Can you work these out from the model? Positions are in its coordinate system, mm. Round coordinates to 2 decimals unless told otherwise and drop trailing zeros. Loops run counter-clockwise (first coordinate to the right, second up) from the corner with the lowest first, then second, coordinate; pieces in that order, holes last. Notation, with made-up numbers: (-25.75, 35.5) - (-10.75, 35.5) arc R21 cw to (-10.75, 47.5) - close; hole circle Ø7 at (-26.75, 42). An arc over 180 degrees is marked (long way). Answer as CSV lines item,"result".
```python
from build123d import *

# Parameters (mm, degrees)
SKETCH1_W           = 14
SKETCH1_H           = 14
BOSS_EXTRUDE2_DEPTH = 1.2
FILLET1_R           = 1
CUT_EXTRUDE2_REACH  = 3.2
SKETCH2_R           = 2.2


with BuildPart() as part:
    # Sketch1 → Boss-Extrude2 (new body)
    with BuildSketch(Plane.XY):
        with BuildLine():
            Line((81.33, -202.9), (79.33, -202.9))
            Line((79.33, -202.9), (76.73, -202.9))
            Line((76.73, -202.9), (76.73, -212.03))
            Line((76.73, -212.03), (76.73, -283.1))
            Line((76.73, -283.1), (79.4, -283.1))
            Line((79.4, -283.1), (81.33, -283.1))
            Line((81.33, -283.1), (81.33, -270.169))
            Line((81.33, -270.169), (95.33, -270.169))
            Line((95.33, -270.169), (95.33, -284.169))
            Line((95.33, -284.169), (81.6, -284.169))
            Line((81.6, -284.169), (81.6, -285.300000001))
            Line((81.6, -285.300000001), (81.6, -288.000000001))
            Line((81.6, -288.000000001), (104.85, -288.000000001))
            Line((104.85, -288.000000001), (113.94, -288.000000001))
            Line((113.94, -288.000000001), (133.73, -288.000000001))
            Line((133.73, -288.000000001), (136.73, -285.000000001))
            Line((136.73, -285.000000001), (152.86, -285.000000001))
            Line((152.86, -285.000000001), (161.94, -285.000000001))
            Line((161.94, -285.000000001), (178.73, -285.000000001))
            Line((178.73, -285.000000001), (195.659492, -289.51666))
            Line((195.659492, -289.51666), (208.778384908, -297.081045818))
            Line((208.778384908, -297.081045818), (210.094127263, -294.801069106))
            Line((210.094127263, -294.801069106), (210.094924986, -294.799686776))
            ThreePointArc((210.094924986, -294.799686776), (211.43094748, -293.774869597), (213.100313224, -293.994924986))
            Line((213.100313224, -293.994924986), (215.397829273, -295.321900182))
            Line((215.397829273, -295.321900182), (225.98, -277))
            Line((225.98, -277), (225.98, -256.415))
            Line((225.98, -256.415), (225.98, -247.025))
            Line((225.98, -247.025), (225.98, -214.605))
            Line((225.98, -214.605), (225.98, -205.215))
            Line((225.98, -205.215), (225.98, -197))
            ThreePointArc((225.98, -197), (224.515534, -193.464466), (220.98, -192))
            Line((220.98, -192), (206.7, -192))
            Line((206.7, -192), (206.7, -194.6))
            ThreePointArc((206.7, -194.6), (204.5, -196.8), (202.3, -194.6))
            Line((202.3, -194.6), (202.3, -192))
            Line((202.3, -192), (179.02, -192))
            Line((179.02, -192), (169.96, -192))
            Line((169.96, -192), (136.73, -192))
            Line((136.73, -192), (133.73, -192))
            Line((133.73, -192), (127.73, -198))
            Line((127.73, -198), (108.89, -198))
            Line((108.89, -198), (99.78, -198))
            Line((99.78, -198), (82.73, -198))
            Line((82.73, -198), (81.53, -198))
            Line((81.53, -198), (81.53, -200.7))
            Line((81.53, -200.7), (81.53, -201.794))
            Line((81.53, -201.794), (95.33, -201.794))
            Line((95.33, -201.794), (95.33, -215.794))
            Line((95.33, -215.794), (81.33, -215.794))
            Line((81.33, -215.794), (81.33, -202.9))
        make_face()
        with Locations((106.43, -277.169)):
            Rectangle(SKETCH1_W, SKETCH1_H, mode=Mode.SUBTRACT)
        with Locations((124.53, -277.169)):
            Rectangle(SKETCH1_W, SKETCH1_H, mode=Mode.SUBTRACT)
        with Locations((88.33, -260.094)):
            Rectangle(SKETCH1_W, SKETCH1_H, mode=Mode.SUBTRACT)
        with Locations((106.43, -260.094)):
            Rectangle(SKETCH1_W, SKETCH1_H, mode=Mode.SUBTRACT)
        with Locations((124.53, -260.094)):
            Rectangle(SKETCH1_W, SKETCH1_H, mode=Mode.SUBTRACT)
        with Locations((142.63, -255.362582)):
            Rectangle(SKETCH1_W, SKETCH1_H, mode=Mode.SUBTRACT)
        with Locations((168.416577, -274.987582)):
            Rectangle(SKETCH1_W, SKETCH1_H, mode=Mode.SUBTRACT)
        Polygon((194.375574468, -286.3230671), (180.8526129, -282.699600468), (184.476079532, -269.1766389), (197.9990411, -272.800105532), align=None, mode=Mode.SUBTRACT)
        Polygon((221.036025826, -278.856733174), (214.036025826, -290.981088826), (201.911670174, -283.981088826), (208.911670174, -271.856733174), align=None, mode=Mode.SUBTRACT)
        with Locations((160.73, -252.987582)):
            Rectangle(SKETCH1_W, SKETCH1_H, mode=Mode.SUBTRACT)
        with Locations((178.83, -255.362582)):
            Rectangle(SKETCH1_W, SKETCH1_H, mode=Mode.SUBTRACT)
        with Locations((196.916577, -257.737582)):
            Rectangle(SKETCH1_W, SKETCH1_H, mode=Mode.SUBTRACT)
        with Locations((215.005, -248.412582)):
            Rectangle(SKETCH1_W, SKETCH1_H, mode=Mode.SUBTRACT)
        with Locations((88.33, -242.994)):
            Rectangle(SKETCH1_W, SKETCH1_H, mode=Mode.SUBTRACT)
        with Locations((106.43, -242.994)):
            Rectangle(SKETCH1_W, SKETCH1_H, mode=Mode.SUBTRACT)
        with Locations((88.33, -225.894)):
            Rectangle(SKETCH1_W, SKETCH1_H, mode=Mode.SUBTRACT)
        with Locations((106.43, -225.894)):
            Rectangle(SKETCH1_W, SKETCH1_H, mode=Mode.SUBTRACT)
        with Locations((124.53, -242.994)):
            Rectangle(SKETCH1_W, SKETCH1_H, mode=Mode.SUBTRACT)
        with Locations((142.63, -238.269)):
            Rectangle(SKETCH1_W, SKETCH1_H, mode=Mode.SUBTRACT)
        with Locations((124.53, -225.894)):
            Rectangle(SKETCH1_W, SKETCH1_H, mode=Mode.SUBTRACT)
        with Locations((142.63, -221.194)):
            Rectangle(SKETCH1_W, SKETCH1_H, mode=Mode.SUBTRACT)
        with Locations((106.43, -208.794)):
            Rectangle(SKETCH1_W, SKETCH1_H, mode=Mode.SUBTRACT)
        with Locations((124.53, -208.794)):
            Rectangle(SKETCH1_W, SKETCH1_H, mode=Mode.SUBTRACT)
        with Locations((142.63, -204.094)):
            Rectangle(SKETCH1_W, SKETCH1_H, mode=Mode.SUBTRACT)
        with Locations((160.73, -235.894)):
            Rectangle(SKETCH1_W, SKETCH1_H, mode=Mode.SUBTRACT)
        with Locations((178.83, -238.269)):
            Rectangle(SKETCH1_W, SKETCH1_H, mode=Mode.SUBTRACT)
        with Locations((160.73, -218.794)):
            Rectangle(SKETCH1_W, SKETCH1_H, mode=Mode.SUBTRACT)
        with Locations((178.83, -221.169)):
            Rectangle(SKETCH1_W, SKETCH1_H, mode=Mode.SUBTRACT)
        with Locations((196.905, -240.644)):
            Rectangle(SKETCH1_W, SKETCH1_H, mode=Mode.SUBTRACT)
        with Locations((196.93, -223.569)):
            Rectangle(SKETCH1_W, SKETCH1_H, mode=Mode.SUBTRACT)
        with Locations((215.005, -231.319)):
            Rectangle(SKETCH1_W, SKETCH1_H, mode=Mode.SUBTRACT)
        with Locations((160.73, -201.694)):
            Rectangle(SKETCH1_W, SKETCH1_H, mode=Mode.SUBTRACT)
        with Locations((178.83, -204.069)):
            Rectangle(SKETCH1_W, SKETCH1_H, mode=Mode.SUBTRACT)
        with Locations((196.93, -206.494)):
            Rectangle(SKETCH1_W, SKETCH1_H, mode=Mode.SUBTRACT)
    extrude(amount=BOSS_EXTRUDE2_DEPTH)

    # Fillet1
    fillet1_edges = [part.edges().sort_by_distance(p)[0] for p in [
        (208.778384908, -297.081045818, 0.6),
        (81.6, -288.000000001, 0.6),
        (81.6, -284.169, 0.6),
        (81.33, -283.1, 0.6),
        (76.73, -283.1, 0.6),
        (76.73, -202.9, 0.6),
        (81.33, -202.9, 0.6),
        (81.53, -201.794, 0.6),
        (81.53, -198, 0.6),
        (202.3, -192, 0.6),
        (206.7, -192, 0.6),
        (215.397829273, -295.321900182, 0.6),
    ]]
    fillet(fillet1_edges, radius=FILLET1_R)

    # Sketch2 → Cut-Extrude2 (cut, up to next)
    with BuildSketch(Plane.XY.offset(1.2), mode=Mode.PRIVATE) as cut_extrude2_sk1:
        with BuildLine():
            Line((153.73, -228.88), (151.68, -228.88))
            ThreePointArc((151.68, -228.88), (152.921660353, -229.263883383), (153.73, -230.281564029))
            Line((153.73, -230.281564029), (153.73, -228.894))
            Line((153.73, -228.894), (153.73, -228.88))
        make_face()
    cut_extrude2_tool1 = extrude(cut_extrude2_sk1.sketch, amount=-CUT_EXTRUDE2_REACH, mode=Mode.PRIVATE) & part.part
    add(cut_extrude2_tool1.solids().sort_by_distance((153.255364, -229.260338, 1.2))[0], mode=Mode.SUBTRACT)
    # Sketch2 → Cut-Extrude2 (cut, up to next)
    with BuildSketch(Plane.XY.offset(1.2), mode=Mode.PRIVATE) as cut_extrude2_sk2:
        with Locations((151.68, -231.08)):
            Circle(SKETCH2_R)
    cut_extrude2_tool2 = extrude(cut_extrude2_sk2.sketch, amount=-CUT_EXTRUDE2_REACH, mode=Mode.PRIVATE) & part.part
    add(cut_extrude2_tool2.solids().sort_by_distance((151.68, -231.08, 1.2))[0], mode=Mode.SUBTRACT)
    # Sketch2 → Cut-Extrude2 (cut, up to next)
    with BuildSketch(Plane.XY.offset(1.2), mode=Mode.PRIVATE) as cut_extrude2_sk3:
        with BuildLine():
            ThreePointArc((153.73, -231.878435971), (152.921660353, -232.896116617), (151.68, -233.28))
            Line((151.68, -233.28), (153.73, -233.28))
            Line((153.73, -233.28), (153.73, -231.878435971))
        make_face()
    cut_extrude2_tool3 = extrude(cut_extrude2_sk3.sketch, amount=-CUT_EXTRUDE2_REACH, mode=Mode.PRIVATE) & part.part
    add(cut_extrude2_tool3.solids().sort_by_distance((153.255364, -232.899662, 1.2))[0], mode=Mode.SUBTRACT)
    # Sketch2 → Cut-Extrude2 (cut, up to next)
    with BuildSketch(Plane.XY.offset(1.2), mode=Mode.PRIVATE) as cut_extrude2_sk4:
        with BuildLine():
            ThreePointArc((151.68, -233.28), (150.438339647, -232.896116617), (149.63, -231.878435971))
            Line((149.63, -231.878435971), (149.63, -233.28))
            Line((149.63, -233.28), (151.68, -233.28))
        make_face()
    cut_extrude2_tool4 = extrude(cut_extrude2_sk4.sketch, amount=-CUT_EXTRUDE2_REACH, mode=Mode.PRIVATE) & part.part
    add(cut_extrude2_tool4.solids().sort_by_distance((150.104636, -232.899662, 1.2))[0], mode=Mode.SUBTRACT)


solid = part.part
```
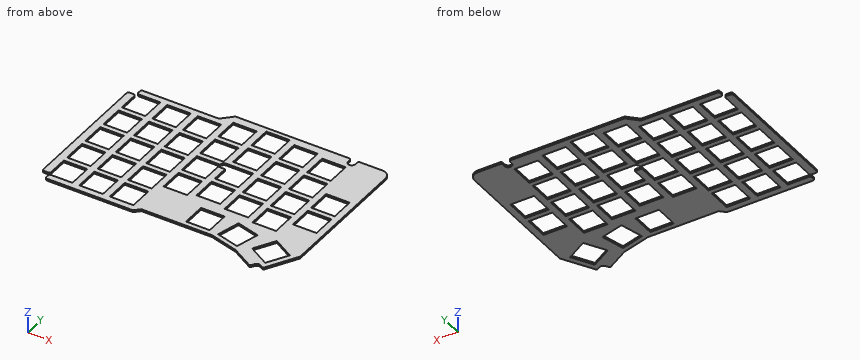
Q1. Imagine slicing it at B-B (y = -221). Count the separate pieces of the cut face and the enclosed holes in it, then the cut area to 3 significant figures.
Checks:
separate pieces,"8"
enclosed holes,"0"
area,"61.5 mm²"
Q2. I'm going to push flat-ended pins straight in: pin 1 Ø5 at (x, y) = (127.5, -279) entering from -Z; pin 2 Ø6 at (x, y) = (210, -202.5) entering from -Z; pin 3 Ø0.6 at (x, z) = (153, 1) entering from -Y; pin 4 Ø0.6 at (y, z) = (-286, 1) entering from -X. Where does each tip first touch, or does it pass through?
Checks:
pin 1,"through"
pin 2,"z = 0"
pin 3,"y = -285"
pin 4,"x = 81.6"
Q3. If I drill on line 1 along X through (y, z) = (-214, 1); line 2 along Y through (x, z) = (156, 0.95); line 3 along Y through (x, z) = (91, 0.5), over which ranges is the centre line in solid material (lowest first)? Write a range as [from, to].
Checks:
line 1,"[76.73, 81.33], [95.33, 99.43], [113.43, 117.53], [131.53, 153.73], [167.73, 225.98]"
line 2,"[-285, -259.99], [-245.99, -242.89], [-228.89, -225.79], [-211.79, -208.69], [-194.69, -192]"
line 3,"[-288, -284.17], [-270.17, -267.09], [-253.09, -249.99], [-235.99, -232.89], [-218.89, -215.79], [-201.79, -198]"
Q4. Imagine slicing it at A-A (x = 159.5). Write out the boundary of the cut face in (y, z).
Checks:
outline,"(-285, 0) - (-259.99, 0) - (-259.99, 1.2) - (-285, 1.2) - close; (-245.99, 0) - (-242.89, 0) - (-242.89, 1.2) - (-245.99, 1.2) - close; (-228.89, 0) - (-225.79, 0) - (-225.79, 1.2) - (-228.89, 1.2) - close; (-211.79, 0) - (-208.69, 0) - (-208.69, 1.2) - (-211.79, 1.2) - close; (-194.69, 0) - (-192, 0) - (-192, 1.2) - (-194.69, 1.2) - close"
Q5. Imagine slicing it at C-C (x = 192.5). Write out the boundary of the cut face in (y, z).
Checks:
outline,"(-288.67, 0) - (-285.82, 0) - (-285.82, 1.2) - (-288.67, 1.2) - close; (-271.33, 0) - (-264.74, 0) - (-264.74, 1.2) - (-271.33, 1.2) - close; (-250.74, 0) - (-247.64, 0) - (-247.64, 1.2) - (-250.74, 1.2) - close; (-233.64, 0) - (-230.57, 0) - (-230.57, 1.2) - (-233.64, 1.2) - close; (-216.57, 0) - (-213.49, 0) - (-213.49, 1.2) - (-216.57, 1.2) - close; (-199.49, 0) - (-192, 0) - (-192, 1.2) - (-199.49, 1.2) - close"
